Geometry: final body of the model. Coordinates: model frame, mm. Face numbers are marked on the shaded views. A direction names the side the tool comes from. Round coordinates to 2 decimals unless told otherwise and drop trailing zeros. Loops run counter-clockwise (first coordinate to the right, second up) from the corner with the lowest first, then second, coordinate; pieces in that order, holes last. Notation, with made-up numbers: M 54.5,23 L 104.5,23 A26 ccw 104.5,48 Z; hole C -6.5,85 d10. An arc over 180 degrees is marked long. Answer as a JSON object with one key per item and string values.
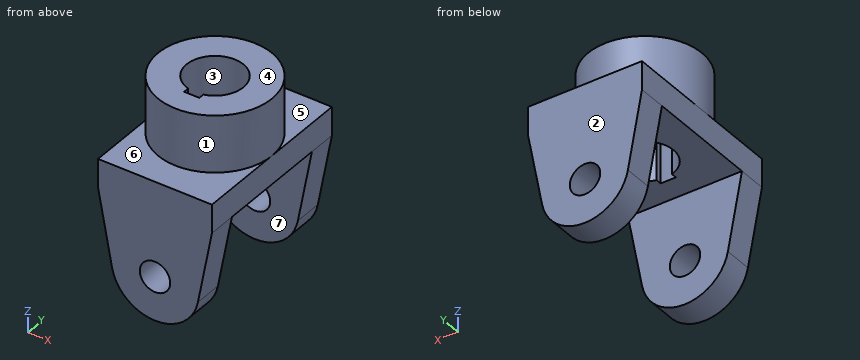
```python
from build123d import *

# Parameters (mm, degrees)
SKETCH2_R           = 8
BOSS_EXTRUDE1_DEPTH = 90
SKETCH3_R           = 30
BOSS_EXTRUDE2_DEPTH = 30
CUT_EXTRUDE1_DEPTH  = 141.032139168
SKETCH5_W           = 58
SKETCH5_H           = 60
CUT_EXTRUDE2_DEPTH  = 135.536240597


with BuildPart() as part:
    # Sketch2 → Boss-Extrude1 (new body)
    with BuildSketch(Plane(origin=(0, 0, 0), x_dir=(1, 0, 0), z_dir=(0, 1, 0))):
        with BuildLine():
            Line((30, -35), (22.602223441, 4.259048664))
            ThreePointArc((22.602223441, 4.259048664), (0, 23), (-22.602223441, 4.259048664))
            Line((-22.602223441, 4.259048664), (-30, -35))
            Line((-30, -35), (-30, -50))
            Line((-30, -50), (30, -50))
            Line((30, -50), (30, -35))
        make_face()
        with Locations(Location((0, 0, 0), (0, 0, 270))):
            Circle(SKETCH2_R, mode=Mode.SUBTRACT)
    extrude(amount=-BOSS_EXTRUDE1_DEPTH)

    # Sketch3 → Boss-Extrude2 (add)
    with BuildSketch(Plane.XY.offset(50)):
        with Locations((0, -45)):
            Circle(SKETCH3_R)
    extrude(amount=BOSS_EXTRUDE2_DEPTH)

    # Sketch4 → Cut-Extrude1 (cut, through all)
    with BuildSketch(Plane.XY.offset(80)):
        with BuildLine():
            Line((-4, -62.456832295), (4, -62.456832295))
            Line((4, -62.456832295), (4, -59.456832295))
            ThreePointArc((4, -59.456832295), (0, -30), (-4, -59.456832295))
            Line((-4, -59.456832295), (-4, -62.456832295))
        make_face()
    extrude(amount=-CUT_EXTRUDE1_DEPTH, mode=Mode.SUBTRACT)

    # Sketch5 → Cut-Extrude2 (cut, through all)
    with BuildSketch(Plane(origin=(30, 0, 0), x_dir=(0, 0, -1), z_dir=(1, 0, 0))):
        with Locations((-6, -45)):
            Rectangle(SKETCH5_W, SKETCH5_H)
    extrude(amount=-CUT_EXTRUDE2_DEPTH, mode=Mode.SUBTRACT)


solid = part.part
```
1) Cut plane A-A on x = 0. Return the cut outline in (y, z).
Geometry results:
{"outline": "M -90,-23 L -75,-23 L -75,-8 L -90,-8 Z; M -90,8 L -75,8 L -75,35 L -62.46,35 L -62.46,80 L -75,80 L -75,50 L -90,50 Z; M -30,35 L -15,35 L -15,8 L 0,8 L 0,50 L -15,50 L -15,80 L -30,80 Z; M -15,-23 L 0,-23 L 0,-8 L -15,-8 Z"}
2) Pull-direction query (X, two-part tool) for the marked faces 1, 2 and 3; classes: +X half, -X half, draft (parallel to the pull), parting line (faces both ways), or undercut.
Geometry results:
{"face 1": "parting line", "face 2": "draft", "face 3": "undercut"}
3) Line query: probe 1 along Y at (x, z) = (17, 1.5); probe 2 along X at (y, z) = (-5, 0); probe 3 along Z at (x, y) = (1.5, -69). Output: solid intervals per line, ascending.
Geometry results:
{"probe 1": "-90 to -75, -15 to 0", "probe 2": "-23.4 to -8, 8 to 23.4", "probe 3": "35 to 80"}
4) Cut plane C-C on z = 1. Return the cut outline in (x, y), and give its area (3 significant figures).
Geometry results:
{"outline": "M -23.59,-90 L -7.94,-90 L -7.94,-75 L -23.59,-75 Z; M -23.59,-15 L -7.94,-15 L -7.94,0 L -23.59,0 Z; M 7.94,-90 L 23.59,-90 L 23.59,-75 L 7.94,-75 Z; M 7.94,-15 L 23.59,-15 L 23.59,0 L 7.94,0 Z", "area": "939 mm2"}
5) Cut plane D-D on z = 68.5. Return the cut outline in (x, y), and give its area (3 significant figures).
Geometry results:
{"outline": "C 0,-45 d60; hole M -4,-62.46 L 4,-62.46 L 4,-59.46 A15 ccw long -4,-59.46 Z", "area": "2,100 mm2"}
6) Cut plane B-B on y = -38. Return the cut outline in (x, z), and give its area (3 significant figures).
Geometry results:
{"outline": "M -30,35 L -13.27,35 L -13.27,80 L -29.17,80 L -29.17,50 L -30,50 Z; M 13.27,35 L 30,35 L 30,50 L 29.17,50 L 29.17,80 L 13.27,80 Z", "area": "1,460 mm2"}
7) First-contact query: pin 1 (6 mm diameter, centred on x = -16, y = -74.5, fed in from +Z); pin 2 (4 mm diameter, centred on x = -0.5, z = 50, fed in from +Y); pin 3 (10 mm diameter, centred on y = -74, z = 6, fed in from +X); pin 4 (1.5 mm diameter, centred on y = -60.5, z = 63, fed in from -X). Flat tips, straight axial feed; report the tip coordinate or a pass-through.
Geometry results:
{"pin 1": "z = 50", "pin 2": "y = 0", "pin 3": "x = 25.46", "pin 4": "x = -26.12"}
8) Set-up query: the marked faces 4, 5, 6 and 7. Return all of +Z, -Z, +X, -X, +Y, -Y with unobstructed straight access to the full face (end or side cutting, diameter ignored); none if empty.
Geometry results:
{"face 4": "+Z, +X, -X, +Y, -Y", "face 5": "+Z, +Y", "face 6": "+Z, -Y", "face 7": "-Z, +X, -X"}
